Design review of the part built by this model. Coordinates are the model's own, in mm. A direction names the side the tool comes from. Give positions to 0.01 mm unless a question says otherwise; leave off trailing zeros. Write each loop counter-clockwise with the first axis right and the second up, starting at its lowest first coordinate (ties: lowest second). Pieces come first, ordered by that corner, then holes.
```python
from build123d import *

# Parameters (mm, degrees)
SKETCH1_R               = 22.5
BOSS_EXTRUDE1_DEPTH     = 60
SKETCH2_R               = 15
CUT_EXTRUDE1_DEPTH      = 12
SKETCH6_W               = 2
SKETCH6_H               = 10
SKETCH7_R               = 22.5
CUT_EXTRUDE2_DEPTH      = 27.5
SKETCH8_R               = 15
CUT_EXTRUDE3_DEPTH      = 27.5
SKETCH9_R               = 2
CUT_EXTRUDE5_DEPTH      = 23.5
CUT_EXTRUDE5_DEPTH_BACK = 23.5
SKETCH10_R              = 15
BOSS_EXTRUDE2_DEPTH     = 32.5
SKETCH11_R              = 3
CUT_EXTRUDE8_DEPTH      = 23.5
CUT_EXTRUDE8_DEPTH_BACK = 23.5
SKETCH12_R              = 3
CUT_EXTRUDE9_DEPTH      = 32.5


with BuildPart() as part:
    # Sketch1 → Boss-Extrude1 (new body)
    with BuildSketch(Plane(origin=(0, 0, 0), x_dir=(1, 0, 0), z_dir=(0, 1, 0))):
        Circle(SKETCH1_R)
    extrude(amount=BOSS_EXTRUDE1_DEPTH)

    # Sketch2 → Cut-Extrude1 (cut)
    with BuildSketch(Plane(origin=(0, 60, 0), x_dir=(1, 0, 0), z_dir=(0, 1, 0))):
        Circle(SKETCH2_R)
    extrude(amount=-CUT_EXTRUDE1_DEPTH, mode=Mode.SUBTRACT)

    # Sketch6 → Cut-Revolve1 (revolve, cut)
    with BuildSketch(Plane.XY):
        with Locations((-21.5, 52.5)):
            Rectangle(SKETCH6_W, SKETCH6_H)
        with Locations((-21.5, 37.5)):
            Rectangle(SKETCH6_W, SKETCH6_H)
        with Locations((-21.5, 22.5)):
            Rectangle(SKETCH6_W, SKETCH6_H)
        with Locations((-21.5, 7.5)):
            Rectangle(SKETCH6_W, SKETCH6_H)
    revolve(axis=Axis((0, 0, 0), (0, 1, 0)), mode=Mode.SUBTRACT)

    # Sketch7 → Cut-Extrude2 (cut)
    with BuildSketch(Plane.XZ):
        Circle(SKETCH7_R)
    extrude(amount=-CUT_EXTRUDE2_DEPTH, mode=Mode.SUBTRACT)

    # Sketch8 → Cut-Extrude3 (cut)
    with BuildSketch(Plane(origin=(0, 48, 0), x_dir=(1, 0, 0), z_dir=(0, 1, 0))):
        Circle(SKETCH8_R)
    extrude(amount=-CUT_EXTRUDE3_DEPTH, mode=Mode.SUBTRACT)

    # Sketch9 → Cut-Extrude5 (cut, two sides)
    with BuildSketch(Plane(origin=(0, 0, 0), x_dir=(0, 0, -1), z_dir=(1, 0, 0))) as cut_extrude5_sk:
        with Locations((0, 52.5)):
            Circle(SKETCH9_R)
    extrude(amount=CUT_EXTRUDE5_DEPTH, mode=Mode.SUBTRACT)
    extrude(cut_extrude5_sk.sketch, amount=-CUT_EXTRUDE5_DEPTH_BACK, mode=Mode.SUBTRACT)

    # Sketch10 → Boss-Extrude2 (add)
    with BuildSketch(Plane(origin=(0, 60, 0), x_dir=(1, 0, 0), z_dir=(0, 1, 0))):
        Circle(SKETCH10_R)
    extrude(amount=-BOSS_EXTRUDE2_DEPTH)

    # Sketch11 → Cut-Extrude8 (cut, two sides)
    with BuildSketch(Plane(origin=(0, 0, 0), x_dir=(0, 0, -1), z_dir=(1, 0, 0))) as cut_extrude8_sk:
        with Locations((0, 52.5)):
            Circle(SKETCH11_R)
    extrude(amount=CUT_EXTRUDE8_DEPTH, mode=Mode.SUBTRACT)
    extrude(cut_extrude8_sk.sketch, amount=-CUT_EXTRUDE8_DEPTH_BACK, mode=Mode.SUBTRACT)

    # Sketch12 → Cut-Extrude9 (cut)
    with BuildSketch(Plane(origin=(0, 60, 0), x_dir=(1, 0, 0), z_dir=(0, 1, 0))):
        Circle(SKETCH12_R)
    extrude(amount=-CUT_EXTRUDE9_DEPTH, mode=Mode.SUBTRACT)


solid = part.part
```
(1) Consider section C-C, the plane z = 11. Give the boundary of the cut face in (x, y), then the cut area to 3 significant figures.
Resolved:
outline: (-19.63, 27.5) - (19.63, 27.5) - (19.63, 32.5) - (17.3, 32.5) - (17.3, 42.5) - (19.63, 42.5) - (19.63, 47.5) - (17.3, 47.5) - (17.3, 57.5) - (19.63, 57.5) - (19.63, 60) - (-19.63, 60) - (-19.63, 57.5) - (-17.3, 57.5) - (-17.3, 47.5) - (-19.63, 47.5) - (-19.63, 42.5) - (-17.3, 42.5) - (-17.3, 32.5) - (-19.63, 32.5) - close
area: 1,180 mm2
(2) Consider section D-D, the plane x = 11.5. Give the boundary of the cut face in (y, z).
Resolved:
outline: (27.5, -19.34) - (32.5, -19.34) - (32.5, -16.97) - (42.5, -16.97) - (42.5, -19.34) - (47.5, -19.34) - (47.5, -16.97) - (57.5, -16.97) - (57.5, -19.34) - (60, -19.34) - (60, 19.34) - (57.5, 19.34) - (57.5, 16.97) - (47.5, 16.97) - (47.5, 19.34) - (42.5, 19.34) - (42.5, 16.97) - (32.5, 16.97) - (32.5, 19.34) - (27.5, 19.34) - close; hole circle Ø6 at (52.5, 0)
(3) To check wall thickness, follow L1, parallel to Y at x = 13.5, z = 16.5; L2, parallel to Z at x = 0, y = 57. State the ranges of each line that lie inside material, in increasing order.
Resolved:
L1: y = 27.5 to 32.5, 42.5 to 47.5, 57.5 to 60
L2: z = -20.5 to -3, 3 to 20.5
(4) Clearance check with flat-ended pins moving along their axes: P1, Ø1, axis at x = -14.5, y = 38, coming from the +Z side (3 decimals); P2, Ø8, axis at x = -17.5, y = 44, coming from the -Z side; P3, Ø4, axis at x = 13.5, y = 45, coming from the -Z side; P4, Ø3.5, axis at x = 0, z = 0, coming from the -Y side. State where each tip first meets the part, or that it passes through.
Resolved:
P1: stops at z = 14.975
P2: stops at z = -18
P3: stops at z = -19.34
P4: passes through
(5) Tool access review of faces 1 (the face through (-9.9, 57.5, -18.2)), 2 (the face through (-3, 40, 0)): name each direction out of +Z, -Z, +X, -X, +Y, -Y from which nothing blocks a thin tool from reaching the whole face with its end or side.
Resolved:
face 1: none
face 2: +Y, -Y
(6) Mouldability with a two-part tool opening along Y and no side actions: class faces 3 (the face through (0, 27.5, -5)), 4 (the face through (-9.9, 32.5, -18.2)), 5 (the face through (10.382, 58.732, 19.961)) as pulls with the +Y half, pulls with the -Y half, needs draft (parallel to the pull), parting line crosses it, or undercut.
Resolved:
face 3: pulls with the -Y half
face 4: undercut
face 5: needs draft
(7) Consider section A-A, the plane x = 18. Give the boundary of the cut face in (y, z).
Resolved:
outline: (27.5, -13.5) - (32.5, -13.5) - (32.5, -9.81) - (42.5, -9.81) - (42.5, -13.5) - (47.5, -13.5) - (47.5, -9.81) - (57.5, -9.81) - (57.5, -13.5) - (60, -13.5) - (60, 13.5) - (57.5, 13.5) - (57.5, 9.81) - (47.5, 9.81) - (47.5, 13.5) - (42.5, 13.5) - (42.5, 9.81) - (32.5, 9.81) - (32.5, 13.5) - (27.5, 13.5) - close; hole circle Ø6 at (52.5, 0)
(8) Consider section B-B, the plane y = 48.5. Give the boundary of the cut face in (x, z).
Resolved:
outline: circle Ø41 at (0, 0); hole circle Ø6 at (0, 0)
